Answer from the drawing. Dimensions are ordinates in mm from the lowest x, y and z of the part. Coordinates: 2 decimals unless noted, no trailing zeros. Loops run counter-clockwise (first coordinate to the right, second up) from the corner with the lowest first, then second, coordinate; pieces in that order, holes last. Notation, with made-up numbers: M -11.75,51 L 25.25,51 A25 cw 25.25,64 Z; hole C 28,61 d11. An arc over 180 degrees is marked long. Put each result on its own line as item: value.
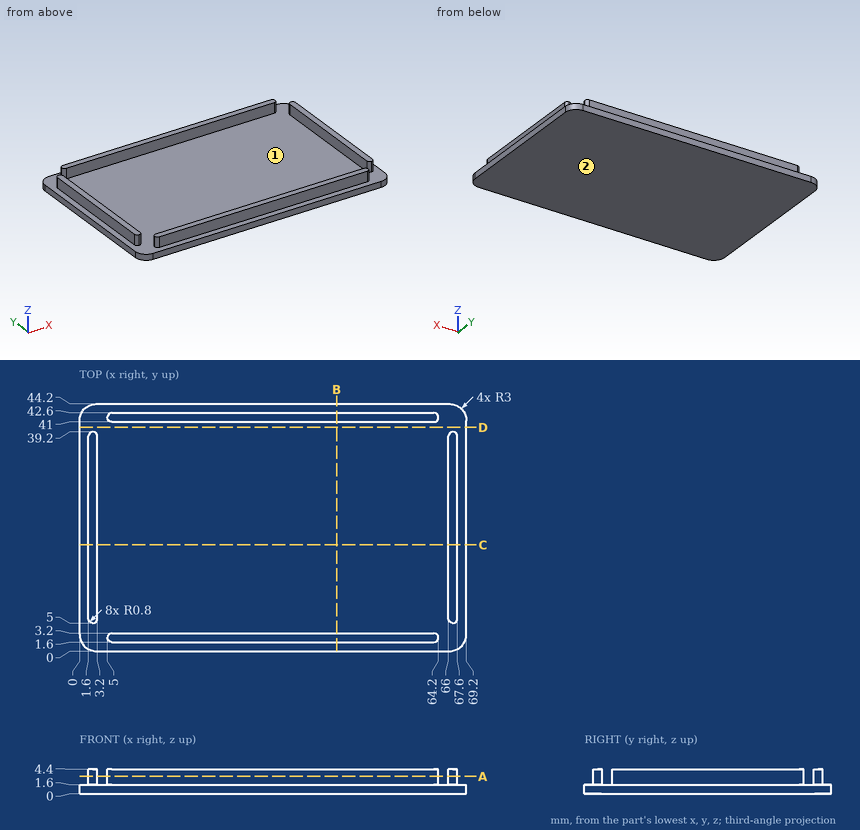
1) Find section C-C, the plane y = 19. Write down the section's boundary in (x, z), plus the area to 3 significant figures.
Answer list:
outline: M 0,0 L 69.2,0 L 69.2,1.6 L 67.6,1.6 L 67.6,4.4 L 66,4.4 L 66,1.6 L 3.2,1.6 L 3.2,4.4 L 1.6,4.4 L 1.6,1.6 L 0,1.6 Z
area: 120 mm^2
2) Find section A-A, the plane z = 3.1. Count the separate pieces of the cut face and the enclosed holes in it, plus the area to 3 significant figures.
Answer list:
separate pieces: 4
enclosed holes: 0
area: 297 mm^2
3) Find section B-B, the plane x = 46. Write down the section's boundary in (y, z), plus the area to 3 significant figures.
Answer list:
outline: M 0,0 L 44.2,0 L 44.2,1.6 L 42.6,1.6 L 42.6,4.4 L 41,4.4 L 41,1.6 L 3.2,1.6 L 3.2,4.4 L 1.6,4.4 L 1.6,1.6 L 0,1.6 Z
area: 79.7 mm^2
4) Find section D-D, the plane y = 40. Write down the section's boundary in (x, z), plus the area to 3 significant figures.
Answer list:
outline: M 0,0 L 69.2,0 L 69.2,1.6 L 0,1.6 Z
area: 111 mm^2
5) Determine the mould class of the marked faces 1 and 2 for opening direction Y: released by +Y, released by -Y, zero draft, split by the parting line, or undercut.
Answer list:
face 1: undercut
face 2: zero draft
6) Given pin 1 Ø1.4 at (y, z) = (23, 3) entering from -X; pin 2 Ø2 at (y, z) = (17, 3.5) entering from +X; pin 3 Ø1.4 at (x, z) = (41, 2.5) entering from -Y, each flat-ended and moving along its own axis, determine where each tip first touches the part or whether it passes through.
Answer list:
pin 1: stops at x = 1.6
pin 2: stops at x = 67.6
pin 3: stops at y = 1.6
7) Straight lines are drawn through the part: line 1 (X direction, y = 24.5, z = 3.15); line 2 (Y direction, x = 32.5, z = 2.6); line 3 (Z direction, x = 38.5, y = 17). For each, find the intervals that lie inside material, in ascending order. Write a range as [from, to].
Answer list:
line 1: x = [1.6, 3.2], [66, 67.6]
line 2: y = [1.6, 3.2], [41, 42.6]
line 3: z = [0, 1.6]
